Source: CAD feature listing. Evaluate the final solid. Frame: model axes, mm. A direction names the side the tool comes from. Coordinates: 2 decimals unless noted, no trailing zeros. Write each loop counter-clockwise with the first axis right and the second up, starting at its lowest first coordinate (ties: lowest second). Pieces come first, ordered by that corner, then holes. Notation, with made-up numbers: (21, -2.75) - (68, -2.75) arc R27 cw to (68, 32.25) - close; hole circle Ø8 at (1, 29.25). An arc over 180 degrees is marked (long way). One line per question, with ' | ' between items.
from build123d import *

# Parameters (mm, degrees)
F0_W     = 372
F0_H     = 240
F1_DEPTH = 9
F2_W     = 9
F2_H     = 12
F3_DEPTH = 9
F4_W     = 12
F4_H     = 9
F5_DEPTH = 9


with BuildPart() as f1:
    # F0 (on Front) → F1 (new body)
    with BuildSketch(Plane.XZ):
        Rectangle(F0_W, F0_H)
    extrude(amount=F1_DEPTH)

    # F2 (on face) → F3 (join, through all)
    with BuildSketch(Plane.XZ.offset(9)):
        with Locations((-190.5, 114)):
            Rectangle(F2_W, F2_H)
        with Locations((-190.5, 90)):
            Rectangle(F2_W, F2_H)
        with Locations((-190.5, 66)):
            Rectangle(F2_W, F2_H)
        with Locations((-190.5, 42)):
            Rectangle(F2_W, F2_H)
        with Locations((-190.5, 18)):
            Rectangle(F2_W, F2_H)
        with Locations((-190.5, -6)):
            Rectangle(F2_W, F2_H)
        with Locations((-190.5, -30)):
            Rectangle(F2_W, F2_H)
        with Locations((-190.5, -54)):
            Rectangle(F2_W, F2_H)
        with Locations((-190.5, -78)):
            Rectangle(F2_W, F2_H)
        with Locations((-190.5, -102)):
            Rectangle(F2_W, F2_H)
        with Locations((190.5, 114)):
            Rectangle(F2_W, F2_H)
        with Locations((190.5, 90)):
            Rectangle(F2_W, F2_H)
        with Locations((190.5, -30)):
            Rectangle(F2_W, F2_H)
        with Locations((190.5, -102)):
            Rectangle(F2_W, F2_H)
        with Locations((190.5, -6)):
            Rectangle(F2_W, F2_H)
        with Locations((190.5, -54)):
            Rectangle(F2_W, F2_H)
        with Locations((190.5, -78)):
            Rectangle(F2_W, F2_H)
        with Locations((190.5, 18)):
            Rectangle(F2_W, F2_H)
        with Locations((190.5, 42)):
            Rectangle(F2_W, F2_H)
        with Locations((190.5, 66)):
            Rectangle(F2_W, F2_H)
    extrude(amount=-F3_DEPTH)

    # F4 (on face) → F5 (join, through all)
    with BuildSketch(Plane.XZ.offset(9)):
        with Locations((0, -124.5)):
            Rectangle(F4_W, F4_H)
        with Locations((24, -124.5)):
            Rectangle(F4_W, F4_H)
        with Locations((48, -124.5)):
            Rectangle(F4_W, F4_H)
        with Locations((72, -124.5)):
            Rectangle(F4_W, F4_H)
        with Locations((96, -124.5)):
            Rectangle(F4_W, F4_H)
        with Locations((120, -124.5)):
            Rectangle(F4_W, F4_H)
        with Locations((144, -124.5)):
            Rectangle(F4_W, F4_H)
        with Locations((168, -124.5)):
            Rectangle(F4_W, F4_H)
        with Locations((-24, -124.5)):
            Rectangle(F4_W, F4_H)
        with Locations((-96, -124.5)):
            Rectangle(F4_W, F4_H)
        with Locations((-120, -124.5)):
            Rectangle(F4_W, F4_H)
        with Locations((-168, -124.5)):
            Rectangle(F4_W, F4_H)
        with Locations((-48, -124.5)):
            Rectangle(F4_W, F4_H)
        with Locations((-144, -124.5)):
            Rectangle(F4_W, F4_H)
        with Locations((-72, -124.5)):
            Rectangle(F4_W, F4_H)
    extrude(amount=-F5_DEPTH)


solid = f1.part
Item 1: Cut plane A-A on z = -92. Return loops of the section in (x, y), and give its area (3 significant figures).
Check sheet entries:
outline: (-186, -9) - (186, -9) - (186, 0) - (-186, 0) - close | area: 3,350 mm²
Item 2: Ray query, line 1 along X through (y, z) = (-4.25, 11.5); line 2 along Z through (x, y) = (84, -3.25). Return the intervals inside material, ascending. Write a range as [from, to].
Check sheet entries:
line 1: [-186, 186] | line 2: [-120, 120]
Item 3: Access query for faces 4 (the face through (-78, -5, -125)), 5 (the face through (195, -5, 114)), 6 (the face through (-186, -4, -90)), 7 (the face through (190, -5, -48)). Directions: +Z, -Z, +X, -X, +Y, -Y. A direction counts if a zero-diameter tool reaches every point of the face in a straight line with its end or side. Return the directions, or none.
Check sheet entries:
face 4: -Z, +Y, -Y | face 5: +Z, -Z, +X, +Y, -Y | face 6: -X, +Y, -Y | face 7: +X, +Y, -Y
Item 4: Pin query (flat end, axial travel): pin 1 Ø4.5 at (x, y) = (58, -4.5) entering from -Z; pin 2 Ø4.5 at (y, z) = (-6.5, -123.5) entering from -X; pin 3 Ø4.5 at (y, z) = (-5, 6.5) entering from +X. Return the tip coordinate at first contact, or that it passes through.
Check sheet entries:
pin 1: z = -120 | pin 2: x = -174 | pin 3: x = 186
Item 5: Mould query, pull axis X, two halves, no side actions, for faces 1 (the face through (-168, -5, -129)), 2 (the face through (174, -5, -125)), 3 (the face through (-66, -5, -125)). Classes: pulls with the +X half, pulls with the -X half, needs draft (parallel to the pull), parting line crosses it, or undercut.
Check sheet entries:
face 1: needs draft | face 2: pulls with the +X half | face 3: undercut
Item 6: Cut plane B-B on x = -85.5. Return loops of the section in (y, z), and give its area (3 significant figures).
Check sheet entries:
outline: (-9, -120) - (0, -120) - (0, 120) - (-9, 120) - close | area: 2,160 mm²
